```python
from build123d import *

# Parameters (mm, degrees)
SKETCH1_W           = 71
SKETCH1_H           = 67
SKETCH1_W_2         = 67
SKETCH1_H_2         = 63
BOSS_EXTRUDE1_DEPTH = 5
SKETCH2_R           = 0.9
CUT_EXTRUDE1_DEPTH  = 121
SKETCH3_R           = 1
CUT_EXTRUDE2_DEPTH  = 90
SKETCH4_W           = 4
SKETCH4_H           = 5
BOSS_EXTRUDE2_DEPTH = 10
SKETCH5_R           = 1
CUT_EXTRUDE3_DEPTH  = 109
SKETCH9_W           = 5.2
SKETCH9_H           = 5
CUT_EXTRUDE6_DEPTH  = 1
SKETCH10_W          = 5.2
SKETCH10_H          = 5
CUT_EXTRUDE7_DEPTH  = 1
SKETCH11_R          = 0.9
CUT_EXTRUDE8_DEPTH  = 81
SKETCH12_R          = 0.9
CUT_EXTRUDE9_DEPTH  = 81


with BuildPart() as part:
    # Sketch1 → Boss-Extrude1 (new body)
    with BuildSketch(Plane(origin=(0, 0, 0), x_dir=(1, 0, 0), z_dir=(0, 1, 0))):
        Rectangle(SKETCH1_W, SKETCH1_H)
        Rectangle(SKETCH1_W_2, SKETCH1_H_2, mode=Mode.SUBTRACT)
    extrude(amount=BOSS_EXTRUDE1_DEPTH)

    # Sketch2 → Cut-Extrude1 (cut)
    with BuildSketch(Plane(origin=(35.5, 0, 0), x_dir=(0, 0, -1), z_dir=(1, 0, 0))):
        with Locations((-6.999701476, 2.591425228)):
            Circle(SKETCH2_R)
        with Locations((7, 2.5)):
            Circle(SKETCH2_R)
    extrude(amount=-CUT_EXTRUDE1_DEPTH, mode=Mode.SUBTRACT)

    # Sketch3 → Cut-Extrude2 (cut)
    with BuildSketch(Plane.XY.offset(33.5)):
        with Locations((0, 2.5)):
            Circle(SKETCH3_R)
    extrude(amount=-CUT_EXTRUDE2_DEPTH, mode=Mode.SUBTRACT)

    # Sketch4 → Boss-Extrude2 (add)
    with BuildSketch(Plane.XY.offset(33.5)):
        with Locations((5.425, 2.5)):
            Rectangle(SKETCH4_W, SKETCH4_H)
        with Locations((-5.428919328, 2.5)):
            Rectangle(SKETCH4_W, SKETCH4_H)
    boss_extrude2 = extrude(amount=BOSS_EXTRUDE2_DEPTH)

    # Mirror1: Boss-Extrude2 across plane
    add(boss_extrude2.mirror(Plane.XY))

    # Sketch5 → Cut-Extrude3 (cut)
    with BuildSketch(Plane.XY.offset(33.5)):
        with Locations((-10.428919328, 2.5)):
            Circle(SKETCH5_R)
        with Locations((10.425, 2.5)):
            Circle(SKETCH5_R)
    extrude(amount=-CUT_EXTRUDE3_DEPTH, mode=Mode.SUBTRACT)

    # Sketch9 → Cut-Extrude6 (cut)
    with BuildSketch(Plane.XY.offset(33.5)):
        with Locations((-27.9, 2.5)):
            Rectangle(SKETCH9_W, SKETCH9_H)
        with Locations((27.9, 2.5)):
            Rectangle(SKETCH9_W, SKETCH9_H)
    cut_extrude6 = extrude(amount=-CUT_EXTRUDE6_DEPTH, mode=Mode.SUBTRACT)

    # Sketch10 → Cut-Extrude7 (cut)
    with BuildSketch(Plane(origin=(35.5, 0, 0), x_dir=(0, 0, -1), z_dir=(1, 0, 0))):
        with Locations((-25.9, 2.5)):
            Rectangle(SKETCH10_W, SKETCH10_H)
        with Locations((25.9, 2.5)):
            Rectangle(SKETCH10_W, SKETCH10_H)
    cut_extrude7 = extrude(amount=-CUT_EXTRUDE7_DEPTH, mode=Mode.SUBTRACT)

    # Mirror2: Cut-Extrude7 across plane
    add(cut_extrude7.mirror(Plane(origin=(0, 0, 0), x_dir=(0, 0, 1), z_dir=(1, 0, 0))), mode=Mode.SUBTRACT)

    # Mirror3: Cut-Extrude6 across plane
    add(cut_extrude6.mirror(Plane.XY), mode=Mode.SUBTRACT)

    # Sketch11 → Cut-Extrude8 (cut)
    with BuildSketch(Plane(origin=(34.5, 0, 0), x_dir=(0, 0, -1), z_dir=(1, 0, 0))):
        with Locations((25.9, 2.5)):
            Circle(SKETCH11_R)
        with Locations((-25.9, 2.5)):
            Circle(SKETCH11_R)
    extrude(amount=-CUT_EXTRUDE8_DEPTH, mode=Mode.SUBTRACT)

    # Sketch12 → Cut-Extrude9 (cut)
    with BuildSketch(Plane.XY.offset(32.5)):
        with Locations((27.9, 2.5)):
            Circle(SKETCH12_R)
        with Locations((-27.9, 2.5)):
            Circle(SKETCH12_R)
    extrude(amount=-CUT_EXTRUDE9_DEPTH, mode=Mode.SUBTRACT)


solid = part.part
```
Design review of the part built by this model. Coordinates are the model's own, in mm. A direction names the side the tool comes from. Coordinates: 2 decimals unless noted, no trailing zeros. Write each loop counter-clockwise with the first axis right and the second up, starting at its lowest first coordinate (ties: lowest second). Pieces come first, ordered by that corner, then holes.
1) Add section C-C (z = 21.5). Write out the cut boundary in (x, y), plus the area to 3 significant figures.
2) Add section A-A (x = 16). Write out the cut boundary in (y, z).
3) Add section B-B (z = -25.9). Write out the cut boundary in (x, y), plus the area to 3 significant figures.
4) Insertion check: pin 1 (2.5 mm diameter, centred on x = -32, y = 2.5, fed in from +Z); pin 2 (2.5 mm diameter, centred on y = 2.5, z = -7, fed in from -X); pin 3 (2.5 mm diameter, centred on y = 3.5, z = 37, fed in from -X); pin 4 (2 mm diameter, centred on x = 2, y = 1.5, fed in from -Z). Each pin has a flat end and moves straight along its axis. Give the tip position at first contact, or say it passes through.
5) Mouldability with a two-part tool opening along Y and no side actions: class faces 1 (the flat face through (0, 1, -31.5)), 2 (the cylindrical face through (11.38, 2.8, 32.51)) as +Y half, -Y half, draft (parallel to the pull), parting line (faces both ways), or undercut.
6) Machinability: for faces 3 (the flat face through (-7.429, 2, 38)), 4 (the flat face through (-28, 4, -32.5)), 5 (the flat face through (33.5, 2, 0)), which of the approach directions +Z, -Z, +X, -X, +Y, -Y give a long, thin tool a straight path to every point of the face, cutting with its end or side? Answer none if there is none.
7) To check wall thickness, follow L1, parallel to Z at x = 24.5, y = 0.3; L2, parallel to X at y = 0.6, z = 10; L3, parallel to Y at x = -27.9, z = -31.85. State the ranges of each line that lie inside material, in increasing order.
8) Add section D-D (x = -27.9). Write out the cut boundary in (y, z), plus the area to 3 significant figures.
Check result:
1. outline: (-35.5, 0) - (-33.5, 0) - (-33.5, 5) - (-35.5, 5) - close; (33.5, 0) - (35.5, 0) - (35.5, 5) - (33.5, 5) - close
1. area: 20.0 mm2
2. outline: (0, -33.5) - (5, -33.5) - (5, -31.5) - (0, -31.5) - close; (0, 31.5) - (5, 31.5) - (5, 33.5) - (0, 33.5) - close
3. outline: (-34.5, 0) - (-33.5, 0) - (-33.5, 1.6) - (-34.5, 1.6) - close; (-34.5, 3.4) - (-33.5, 3.4) - (-33.5, 5) - (-34.5, 5) - close; (33.5, 0) - (34.5, 0) - (34.5, 1.6) - (33.5, 1.6) - close; (33.5, 3.4) - (34.5, 3.4) - (34.5, 5) - (33.5, 5) - close
3. area: 6.40 mm2
4. pin 1: stops at z = 33.5
4. pin 2: stops at x = -35.5
4. pin 3: stops at x = -7.43
4. pin 4: stops at z = -33.5
5. face 1: draft
5. face 2: undercut
6. face 3: +Z, -X, +Y, -Y
6. face 4: -Z, +Y, -Y
6. face 5: +Y, -Y
7. L1: z = -33.5 to -31.5, 31.5 to 33.5
7. L2: x = -35.5 to -33.5, 33.5 to 35.5
7. L3: y = 0 to 1.6, 3.4 to 5
8. outline: (0, -32.5) - (1.6, -32.5) - (1.6, -31.5) - (0, -31.5) - close; (0, 31.5) - (1.6, 31.5) - (1.6, 32.5) - (0, 32.5) - close; (3.4, -32.5) - (5, -32.5) - (5, -31.5) - (3.4, -31.5) - close; (3.4, 31.5) - (5, 31.5) - (5, 32.5) - (3.4, 32.5) - close
8. area: 6.40 mm2
